```python
from build123d import *

# Parameters (mm, degrees)
SKETCH1_W           = 7.5
SKETCH1_H           = 7.5
BOSS_EXTRUDE1_DEPTH = 13
SKETCH2_R           = 1.25
CUT_EXTRUDE1_DEPTH  = 10
SKETCH3_R           = 1.25
CUT_EXTRUDE2_DEPTH  = 10


with BuildPart() as part:
    # Sketch1 → Boss-Extrude1 (new body)
    with BuildSketch(Plane(origin=(0, 0, 0), x_dir=(1, 0, 0), z_dir=(0, 1, 0))):
        Rectangle(SKETCH1_W, SKETCH1_H)
    extrude(amount=BOSS_EXTRUDE1_DEPTH)

    # Sketch2 → Cut-Extrude1 (cut)
    with BuildSketch(Plane(origin=(0, 0, -3.75), x_dir=(-1, 0, 0), z_dir=(0, 0, -1))):
        with Locations((0, 4.053058834)):
            Circle(SKETCH2_R)
    extrude(amount=-CUT_EXTRUDE1_DEPTH, mode=Mode.SUBTRACT)

    # Sketch3 → Cut-Extrude2 (cut)
    with BuildSketch(Plane(origin=(3.75, 0, 0), x_dir=(0, 0, -1), z_dir=(1, 0, 0))):
        with Locations((0, 9)):
            Circle(SKETCH3_R)
    extrude(amount=-CUT_EXTRUDE2_DEPTH, mode=Mode.SUBTRACT)


solid = part.part
```
Geometry check sheet. Reference: the model listing, model coordinates, mm. Coordinates: 2 decimals unless noted, no trailing zeros. Order: outer loops, then holes, each group sorted by start corner. A loop starts at its lowest first (then second) coordinate and runs counter-clockwise, first axis right, second up.
Item 1: Depth check by flat-ended pin: pin 1 (2 mm diameter, centred on x = 0, y = 4.05, fed in from -Z) (3 decimals). Enter the tip coordinate at first touch or a pass-through.
Item 2: Section check D-D (x = -2.25). Enter the section's corners in (y, z), plus the area to 3 significant figures.
Item 3: Scan lines: line 1 along Y through (x, z) = (0, -1.75); line 2 along Y through (x, z) = (-1.5, 0); line 3 along Y through (x, z) = (-1, 0.75). Record each from-to range of solid material in increasing order.
Item 4: Mould release check, pull along Z, two halves, no side actions. Record for faces 1 (the flat face through (0, 6, -3.75)), 2 (the flat face through (-3.75, 6, 0)), 3 (the cylindrical face through (0.05, 10.24, 0.16)): released by +Z, released by -Z, zero draft, split by the parting line, or undercut.
Item 5: Section check B-B (z = 0.25). Enter the section's corners in (x, y).
Item 6: Section check C-C (y = 10). Enter the section's corners in (x, z), plus the area to 3 significant figures.
Item 7: Section check A-A (x = 0). Enter the section's corners in (y, z), plus the area to 3 significant figures.
Check sheet entries:
1. pin 1: passes through
2. outline: (0, -3.75) - (13, -3.75) - (13, 3.75) - (0, 3.75) - close; hole circle Ø2.5 at (9, 0)
2. area: 92.6 mm2
3. line 1: y = 0 to 2.8, 5.3 to 13
3. line 2: y = 0 to 7.75, 10.25 to 13
3. line 3: y = 0 to 3.3, 4.8 to 8, 10 to 13
4. face 1: released by -Z
4. face 2: zero draft
4. face 3: undercut
5. outline: (-3.75, 0) - (3.75, 0) - (3.75, 7.78) - (-3.75, 7.78) - close; (-3.75, 10.22) - (3.75, 10.22) - (3.75, 13) - (-3.75, 13) - close; hole circle Ø2.5 at (0, 4.05)
6. outline: (-3.75, -3.75) - (3.75, -3.75) - (3.75, -0.75) - (-3.75, -0.75) - close; (-3.75, 0.75) - (3.75, 0.75) - (3.75, 3.75) - (-3.75, 3.75) - close
6. area: 45.0 mm2
7. outline: (0, -3.75) - (2.8, -3.75) - (2.8, 3.75) - (0, 3.75) - close; (5.3, -3.75) - (13, -3.75) - (13, 3.75) - (5.3, 3.75) - close; hole circle Ø2.5 at (9, 0)
7. area: 73.8 mm2
